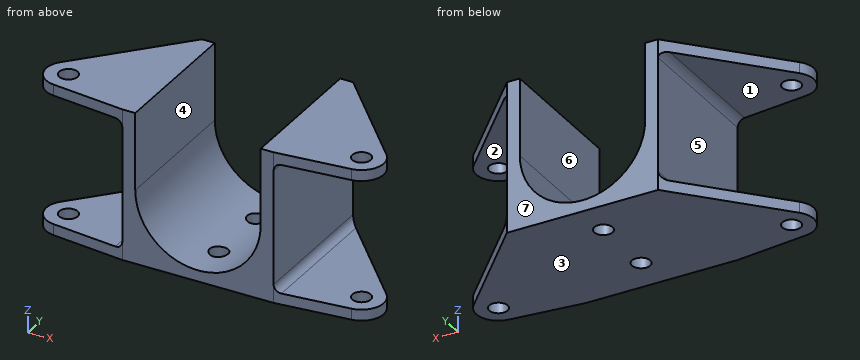
```python
from build123d import *

# Parameters (mm, degrees)
BOSS_EXTRUDE1_DEPTH     = 41
SKETCH3_W               = 25.226628976
SKETCH3_H               = 35
CUT_EXTRUDE2_DEPTH      = 39
CUT_EXTRUDE2_DEPTH_BACK = 1
CUT_EXTRUDE3_DEPTH      = 39
SKETCH5_R               = 2.5
CUT_EXTRUDE4_DEPTH      = 42
SKETCH6_R               = 2.5
CUT_EXTRUDE5_DEPTH      = 42.0000001
FILLET1_R               = 2


with BuildPart() as part:
    # Sketch1 → Boss-Extrude1 (new body)
    with BuildSketch(Plane.XY):
        with BuildLine():
            Line((-20.5, 0), (-40.380779843, 2.180502889))
            ThreePointArc((-40.380779843, 2.180502889), (-45.342396797, 6.03211956), (-44.149663567, 12.198964882))
            Line((-44.149663567, 12.198964882), (-20.5, 38))
            Line((-20.5, 38), (20.5, 38))
            Line((20.5, 38), (44.149663567, 12.198964882))
            ThreePointArc((44.149663567, 12.198964882), (45.342396797, 6.03211956), (40.380779843, 2.180502889))
            Line((40.380779843, 2.180502889), (20.5, 0))
            Line((20.5, 0), (-20.5, 0))
        make_face()
    extrude(amount=BOSS_EXTRUDE1_DEPTH)

    # Sketch3 → Cut-Extrude2 (cut, two sides)
    with BuildSketch(Plane(origin=(0, 0, 0), x_dir=(1, 0, 0), z_dir=(0, 1, 0))) as cut_extrude2_sk:
        with Locations((33.113314488, -20.5)):
            Rectangle(SKETCH3_W, SKETCH3_H)
        with Locations((-33.113314488, -20.5)):
            Rectangle(SKETCH3_W, SKETCH3_H)
    extrude(amount=CUT_EXTRUDE2_DEPTH, mode=Mode.SUBTRACT)
    extrude(cut_extrude2_sk.sketch, amount=-CUT_EXTRUDE2_DEPTH_BACK, mode=Mode.SUBTRACT)

    # Sketch4 → Cut-Extrude3 (cut, through all)
    with BuildSketch(Plane.XZ):
        with BuildLine():
            Line((-17, 20), (-17, 41))
            Line((-17, 41), (17, 41))
            Line((17, 41), (17, 20))
            ThreePointArc((17, 20), (0, 3), (-17, 20))
        make_face()
    extrude(amount=-CUT_EXTRUDE3_DEPTH, mode=Mode.SUBTRACT)

    # Sketch5 → Cut-Extrude4 (cut, through all)
    with BuildSketch(Plane(origin=(0, 0, 0), x_dir=(-1, 0, 0), z_dir=(0, 0, -1))):
        with Locations((0, 28)):
            Circle(SKETCH5_R)
        with Locations((0, 10)):
            Circle(SKETCH5_R)
    extrude(amount=-CUT_EXTRUDE4_DEPTH, mode=Mode.SUBTRACT)

    # Sketch6 → Cut-Extrude5 (cut, through all)
    with BuildSketch(Plane.XY.offset(41)):
        with Locations((-39.726628976, 8.144736842)):
            Circle(SKETCH6_R)
    cut_extrude5 = extrude(amount=-CUT_EXTRUDE5_DEPTH, mode=Mode.SUBTRACT)

    # Mirror1: Cut-Extrude5 across plane
    add(cut_extrude5.mirror(Plane(origin=(0, 0, 0), x_dir=(0, 0, 1), z_dir=(1, 0, 0))), mode=Mode.SUBTRACT)

    # Fillet1
    fillet1_edges = [part.edges().sort_by_distance(p)[0] for p in [
        (20.5, 19, 3),
        (20.5, 19, 38),
        (-20.5, 19, 38),
        (-20.5, 19, 3),
    ]]
    fillet(fillet1_edges, radius=FILLET1_R)


solid = part.part
```
Could you check a few things on this model? Use its own coordinates, in mm. Face numbers are marked on the shaded views. A direction names the side the tool comes from. Give positions to 0.01 mm unless a question says otherwise; leave off trailing zeros. Loops run counter-clockwise (first coordinate to the right, second up) from the corner with the lowest first, then second, coordinate; pieces in that order, holes last. Notation, with made-up numbers: (-25, 54.5) - (5, 54.5) arc R27 ccw to (5, 82.5) - close; hole circle Ø2 at (75.5, -34). An arc over 180 degrees is marked (long way). Use one line per item in the form item = value.
1. Thinking about a two-plate mould opening in X: for the marked faces 4, 5, 6 and 7, which applies, released by +X, released by -X, zero draft, split by the parting line, or undercut?
Response values:
face_4 = undercut
face_5 = released by -X
face_6 = undercut
face_7 = zero draft
2. I want a section at D-D (x = -29). Please give me the cut outline in (y, z).
Response values:
outline = (0.93, 0) - (28.73, 0) - (28.73, 3) - (0.93, 3) - close; (0.93, 38) - (28.73, 38) - (28.73, 41) - (0.93, 41) - close
3. I need wall thicknesses on probe 1 along Y at (x, z) = (0, 2.05); probe 2 along X at (y, z) = (10, 1); probe 3 along X at (y, z) = (36.5, 21). Which ranges of each line are inside material? Lowest first, please.
Response values:
probe_1 = 0 to 7.5, 12.5 to 25.5, 30.5 to 38
probe_2 = -45.43 to -41.4, -38.05 to -2.5, 2.5 to 38.05, 41.4 to 45.43
probe_3 = -20.5 to -17, 17 to 20.5
4. On a 3-axis mill with a long thin cutter (end or side, diameter ignored), from which of +Z, -Z, +X, -X, +Y, -Y can I reach the whole of each face in a straight line? I mean the marked faces 1, 2 and 3. Say none if no direction works.
Response values:
face_1 = -X, +Y, -Y
face_2 = +X, +Y, -Y
face_3 = -Z, +X, -X, +Y, -Y
5. I'm going to push flat-ended pins straight in: pin 1 Ø9.5 at (y, z) = (25.5, 14) entering from -X; pin 2 Ø4 at (x, y) = (39.73, 8.14) entering from +Z; pin 3 Ø1.5 at (x, y) = (12, 7.5) entering from +Z; pin 4 Ø1 at (y, z) = (13, 36.5) entering from -X. Where does each tip first touch, or does it pass through?
Response values:
pin_1 = -20.5
pin_2 = through
pin_3 = 8.76
pin_4 = -20.77
6. I want a section at B-B (x = 0). Please give me the cut outline in (y, z).
Response values:
outline = (0, 0) - (7.5, 0) - (7.5, 3) - (0, 3) - close; (12.5, 0) - (25.5, 0) - (25.5, 3) - (12.5, 3) - close; (30.5, 0) - (38, 0) - (38, 3) - (30.5, 3) - close
7. I want a section at A-A (z = 23.5). Please give me the cut outline in (x, y).
Response values:
outline = (-20.5, 0) - (-17, 0) - (-17, 38) - (-20.5, 38) - close; (17, 0) - (20.5, 0) - (20.5, 38) - (17, 38) - close
8. I want a section at C-C (y = 28). Please give me the cut outline in (x, z), and give its area (3 significant figures).
Response values:
outline = (-29.67, 0) - (-2.5, 0) - (-2.5, 3.18) arc R17 cw to (-17, 20) - (-17, 41) - (-29.67, 41) - (-29.67, 38) - (-22.5, 38) arc R2 cw to (-20.5, 36) - (-20.5, 5) arc R2 cw to (-22.5, 3) - (-29.67, 3) - close; (2.5, 0) - (29.67, 0) - (29.67, 3) - (22.5, 3) arc R2 cw to (20.5, 5) - (20.5, 36) arc R2 cw to (22.5, 38) - (29.67, 38) - (29.67, 41) - (17, 41) - (17, 20) arc R17 cw to (2.5, 3.18) - close
area = 611 mm²
